```python
from build123d import *

# Parameters (mm, degrees)
F3_R      = 15
F1_R      = 50
F4_FACE_R = 15
F6_R      = 15


with BuildPart() as f4:
    # F3 (on offset) → F4 section 0
    with BuildSketch(Plane.XY.offset(-30)):
        Circle(F3_R)
    # F1 (on offset) → F4 section 1
    with BuildSketch(Plane.XY.offset(-70)):
        Circle(F1_R)
    loft()

    # F4_face (on face) → F7 section 0
    with BuildSketch(Plane.XY.offset(-30)):
        Circle(F4_FACE_R)
    # F6 (on offset) → F7 section 1
    with BuildSketch(Plane.XY):
        Circle(F6_R)
    loft()

    # F8 (on Front) → F9 (revolve)
    with BuildSketch(Plane.XZ):
        with BuildLine():
            Line((0, 0), (0, 100.507477))
            Line((0, 100.507477), (-66.673411, 100.507477))
            Line((-66.673411, 100.507477), (-66.673411, 50))
            ThreePointArc((-66.673411, 50), (-52.02875, 14.644661), (-16.673411, 0))
            Line((-16.673411, 0), (0, 0))
        make_face()
    revolve(axis=Axis((0, 0, 50.253739), (0, 0, -1)))


solid = f4.part
```
Here's how the part is built. I have some questions about the finished solid (model axes, mm). A direction names the side the tool comes from. Coordinates: 2 decimals unless noted, no trailing zeros. Order: outer loops, then holes, each group sorted by start corner. A loop starts at its lowest first (then second) coordinate and runs counter-clockwise, first axis right, second up.
Item 1: Thinking about a two-plate mould opening in Z: for faces 1 (the face through (-1, 1, 100.507)), 2 (the face through (-1, 1, -70)), 3 (the face through (-17.17, 0.76, -32.5)), which applies, pulls with the +Z half, pulls with the -Z half, needs draft (parallel to the pull), parting line crosses it, or undercut?
Response values:
face 1: pulls with the +Z half
face 2: pulls with the -Z half
face 3: undercut
Item 2: If we section it at B-B, the plane z = 59: List the corners of the cut face in (x, y) for me, then the cut area to 3 significant figures.
Response values:
outline: circle Ø133.35 at (0, 0)
area: 14,000 mm2
Item 3: I'm going to push flat-ended pins straight in: pin 1 Ø2 at (y, z) = (6.5, 68) entering from +X; pin 2 Ø1 at (x, z) = (22, -43) entering from -Y; pin 3 Ø1.5 at (y, z) = (4, 8.5) entering from +X. Where does each tip first touch, or does it pass through?
Response values:
pin 1: stops at x = 66.45
pin 2: stops at y = -15.6
pin 3: stops at x = 45.47
Item 4: I need wall thicknesses on probe 1 along Z at (x, y) = (43, -10); probe 2 along Z at (x, y) = (43, -10.5); probe 3 along Z at (x, y) = (-23, -49.5). Which ranges of each line are inside material? Lowest first, please.
Response values:
probe 1: z = -70 to -63.31, 8.22 to 100.51
probe 2: z = -70 to -63.44, 8.3 to 100.51
probe 3: z = 17.4 to 100.51
Item 5: If we section it at A-A, the plane z = -19: List the corners of the cut face in (x, y) for me.
Response values:
outline: circle Ø30 at (0, 0)
Item 6: Which directions (+Z, -Z, +X, -X, +Y, -Y) give clear straight access to the entire face, cutting with the end or side of a thin tool? Please do faces 4 (the face through (52.91, -40.57, 74.9)), 5 (the face through (14, 6, 0)).
Response values:
face 4: +Z, -Z
face 5: none
